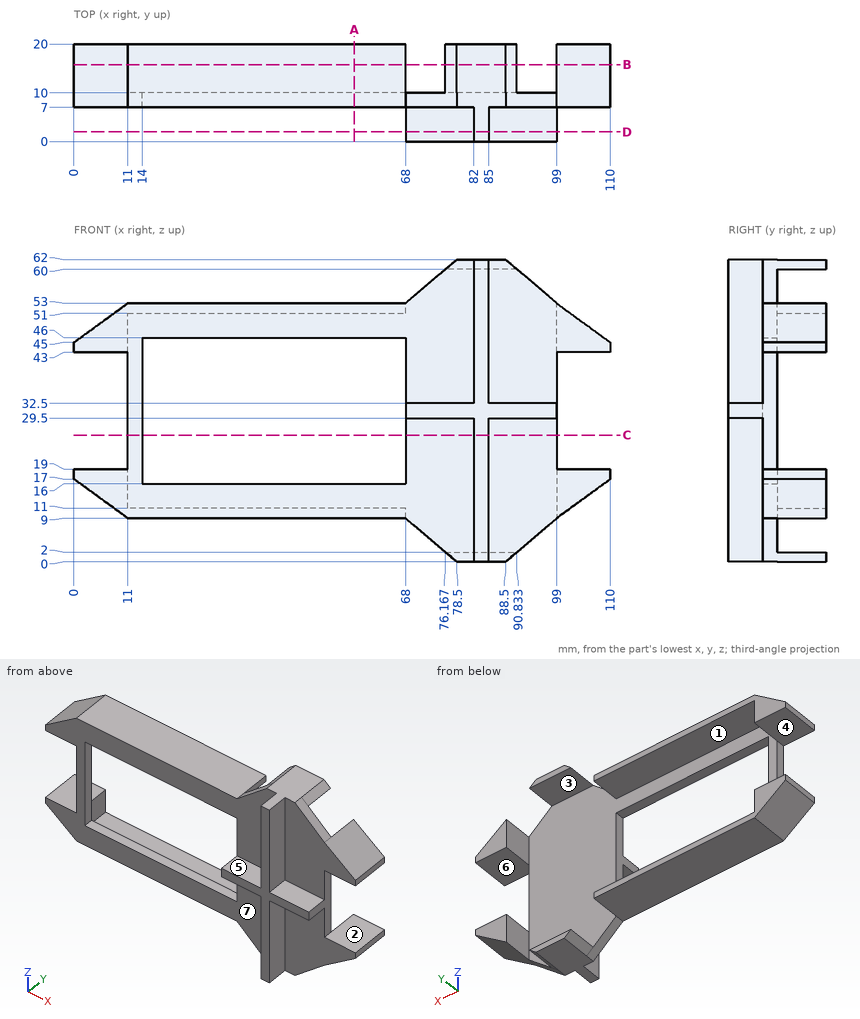
For this review, use the dimensioned drawing (mm, ordinates from the lowest corner) and the shaded views. A direction names the side the tool comes from. Give positions to 0.01 mm unless a question says otherwise; leave off trailing zeros. Order: outer loops, then holes, each group sorted by start corner. A loop starts at its lowest first (then second) coordinate and runs counter-clockwise, first axis right, second up. Notation, with made-up numbers: (-27.5, 26.5) - (5.5, 26.5) arc R24 cw to (5.5, 42.5) - close; hole circle Ø10 at (88.25, -22.5). An arc over 180 degrees is marked (long way). Use a Markdown table: item, result. Add a question column.
(1) Add section C-C on z = 26. Give the boundary of the cut face in (x, y).
(2) Clearance check with flat-ended pins moving along their axes: P1, Ø1, axis at x = 64.5, z = 49, coming from the -Y side; P2, Ø11, axis at x = 52, y = 14.5, coming from the -Z side; P3, Ø3.5, axis at x = 94, y = 5, coming from the -Z side. State where each tip first meets the part, or that it passes through.
(3) Wall thickness on probe 1 along Z at (x, y) = (47.5, 9.5); probe 2 along Z at (x, y) = (20, 15.5); probe 3 along X at (y, z) = (3.5, 14): over which ranges is each line inside the solid? List them lowest first. Write a range as [from, to].
(4) Mouldability with a two-part tool opening along Z and no side actions: class the marked faces 5, 6 and 7 as +Z half, -Z half, draft (parallel to the pull), parting line (faces both ways), or undercut.
(5) Add section A-A on x = 57.5. Give the boundary of the cut face in (y, z).
(6) Machinability: for the marked faces 1, 2, 3 and 4, which of the approach directions +Z, -Z, +X, -X, +Y, -Y give a long, thin tool a straight path to every point of the face, cutting with its end or side? Answer none if there is none.
(7) Add section B-B on y = 15.75. Give the number of separate pieces and of enclosed holes in the cut face.
(8) Add section D-D on y = 2. Give the boundary of the cut face in (x, z), then the cut area to 3 significant figures.
Report:
| question | item | result |
|---|---|---|
| 1 | outline | (11, 7) - (14, 7) - (14, 10) - (11, 10) - close; (68, 7) - (82, 7) - (82, 0) - (85, 0) - (85, 7) - (99, 7) - (99, 10) - (68, 10) - close |
| 2 | P1 | stops at y = 7 |
| 2 | P2 | stops at z = 9 |
| 2 | P3 | stops at z = 29.5 |
| 3 | probe 1 | z = [9, 16], [46, 53] |
| 3 | probe 2 | z = [9, 11], [51, 53] |
| 3 | probe 3 | x = [82, 85] |
| 4 | face 5 | +Z half |
| 4 | face 6 | undercut |
| 4 | face 7 | draft |
| 5 | outline | (7, 9) - (20, 9) - (20, 11) - (10, 11) - (10, 16) - (7, 16) - close; (7, 46) - (10, 46) - (10, 51) - (20, 51) - (20, 53) - (7, 53) - close |
| 6 | face 1 | +Y |
| 6 | face 2 | +X, +Y, -Y |
| 6 | face 3 | +X, -X, +Y |
| 6 | face 4 | -X, +Y, -Y |
| 7 | separate pieces | 6 |
| 7 | enclosed holes | 0 |
| 8 | outline | (68, 29.5) - (82, 29.5) - (82, 0) - (85, 0) - (85, 29.5) - (99, 29.5) - (99, 32.5) - (85, 32.5) - (85, 62) - (82, 62) - (82, 32.5) - (68, 32.5) - close |
| 8 | area | 270 mm² |
